Input: dimensioned drawing with shaded views. Units: mm. Origin: part minimum x, y, z. A direction names the side the tool comes from. Round coordinates to 2 decimals unless told otherwise and drop trailing zeros. Loops run counter-clockwise (first coordinate to the right, second up) from the corner with the lowest first, then second, coordinate; pieces in that order, holes last.
1) Section A-A, the plane y = 3. Return loops of the section in (x, z).
2) Ray query, line 1 along Y through (x, z) = (3.1, 6.25); line 2 along Z through (x, y) = (2.65, 2.8); line 3 along Z through (x, y) = (1, 1.35). Return the intervals inside material, ascending.
3) Section C-C, the plane z = 2. Return loops of the section in (x, y).
4) Section D-D, the plane y = 2.05. Return loops of the section in (x, z).
5) First-contact query: pin 1 (2 mm diameter, centred on x = 3, z = 15, fed in from +Y); pin 2 (1 mm diameter, centred on y = 3.5, z = 16, fed in from +X); pin 3 (0.5 mm diameter, centred on y = 3.5, z = 0.5, fed in from +X). Flat tips, straight axial feed; report the tip coordinate or a pass-through.
6) Access query for the marked faces 1 and 2. Directions: +Z, -Z, +X, -X, +Y, -Y. A direction counts if a zero-diameter tool reaches every point of the face in a straight line with its end or side. Return the directions, or none.
7) Section B-B, the plane x = 3. Return loops of the section in (y, z).
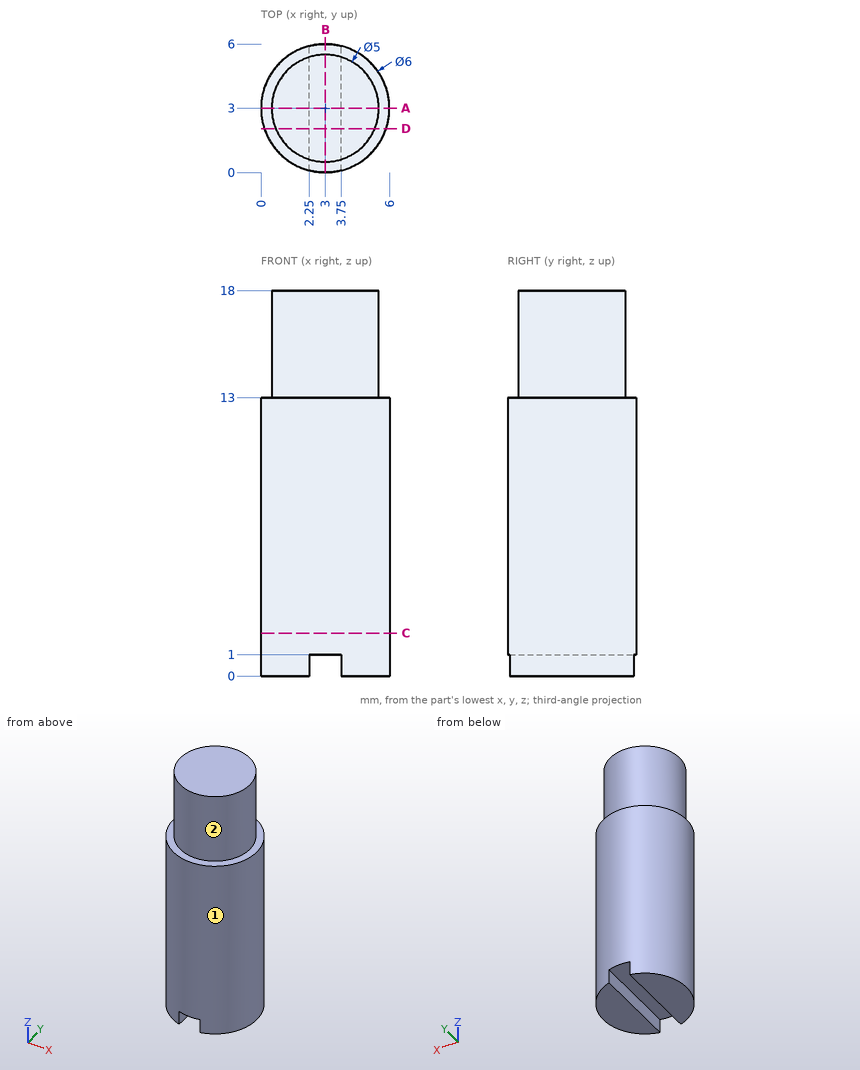
Final values:
1. outline: (0, 0) - (2.25, 0) - (2.25, 1) - (3.75, 1) - (3.75, 0) - (6, 0) - (6, 13) - (5.5, 13) - (5.5, 18) - (0.5, 18) - (0.5, 13) - (0, 13) - close
2. line 1: y = 0 to 6
2. line 2: z = 1 to 18
2. line 3: z = 0 to 13
3. outline: circle Ø6 at (3, 3)
4. outline: (0.15, 0) - (2.25, 0) - (2.25, 1) - (3.75, 1) - (3.75, 0) - (5.85, 0) - (5.85, 13) - (5.31, 13) - (5.31, 18) - (0.69, 18) - (0.69, 13) - (0.15, 13) - close
5. pin 1: stops at y = 5.5
5. pin 2: stops at x = 5.5
5. pin 3: stops at x = 5.99
6. face 1: +Z, -Z
6. face 2: +Z
7. outline: (0, 1) - (6, 1) - (6, 13) - (5.5, 13) - (5.5, 18) - (0.5, 18) - (0.5, 13) - (0, 13) - close
